Source: CAD feature listing. Evaluate the final solid. Frame: model axes, mm. Face numbers are marked on the shaded views. A direction names the side the tool comes from. Coordinates: 2 decimals unless noted, no trailing zeros. Loops run counter-clockwise (first coordinate to the right, second up) from the corner with the lowest first, then second, coordinate; pieces in that order, holes last.
Item 1: Line query: probe 1 along Y at (x, z) = (-23, 19); probe 2 along X at (y, z) = (54.5, 16.5); probe 3 along Z at (x, y) = (23, 43) (3 decimals). Output: solid intervals per line, ascending.
Item 2: Section query A-A, the plane z = 56.5. Return the cut outline in (x, y).
Item 3: Pull-direction query (X, two-part tool) for the marked faces 1, 2 and 3; classes: +X half, -X half, draft (parallel to the pull), parting line (faces both ways), or undercut.
Item 4: Section query C-C, the plane z = 19.05. Return the cut outline in (x, y), then the cut area to 3 significant figures.
Item 5: Reachability of the marked faces 4 and 5 from +Z, -Z, +X, -X, +Y, -Y: full face, straight path, thin tool, end or side. Return the list, or none.
Item 6: Pin query (flat end, axial travel): pin 1 Ø5 at (x, y) = (-11.5, 40) entering from -Z (3 decimals); pin 2 Ø12 at (y, z) = (19, 66.5) entering from -X; pin 3 Ø6 at (x, y) = (31.5, 56.5) entering from -Z. Return the tip coordinate at first contact, or that it passes through.
Item 7: Section query B-B, the plane y = 31.75. State how many separate pieces and enclosed holes the cut face has, then the cut area to 3 significant figures.
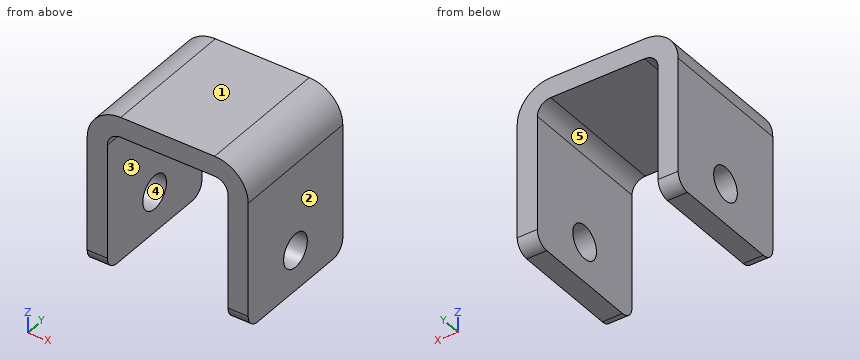
```python
from build123d import *

# Parameters (mm, degrees)
F0_W     = 76.2
F0_H     = 76.2
F1_DEPTH = 63.5
F2_T     = -9.525
F3_R     = 6.35
F4_R     = 15.875
F5_R     = 7.9375
F6_DEPTH = 76.201
F7_R     = 6.35


with BuildPart() as f1:
    # F0 (on Front) → F1 (new body)
    with BuildSketch(Plane.XZ):
        with Locations((7.4331681192, 38.1)):
            Rectangle(F0_W, F0_H)
    extrude(amount=-F1_DEPTH)

    # F2
    f2_openings = [f1.faces().sort_by_distance(p)[0] for p in [
        (7.433168, 0, 38.1),
        (7.433168, 31.75, 0),
        (7.433168, 63.5, 38.1),
    ]]
    offset(amount=F2_T, openings=f2_openings)

    # F3
    f3_edges = [f1.edges().sort_by_distance(p)[0] for p in [
        (-21.141832, 31.75, 66.675),
        (36.008168, 31.75, 66.675),
    ]]
    fillet(f3_edges, radius=F3_R)

    # F4
    f4_edges = [f1.edges().sort_by_distance(p)[0] for p in [
        (-30.666832, 31.75, 76.2),
        (45.533168, 31.75, 76.2),
    ]]
    fillet(f4_edges, radius=F4_R)

    # F5 (on face) → F6 (cut, through all)
    with BuildSketch(Plane.YZ.offset(45.5331681192)):
        with Locations((31.75, 19.05)):
            Circle(F5_R)
    extrude(amount=-F6_DEPTH, mode=Mode.SUBTRACT)

    # F7
    f7_edges = [f1.edges().sort_by_distance(p)[0] for p in [
        (-25.904332, 0, 0),
        (40.770668, 0, 0),
        (-25.904332, 63.5, 0),
        (40.770668, 63.5, 0),
    ]]
    fillet(f7_edges, radius=F7_R)


solid = f1.part
```
Verdict:
1. probe 1: y = 0 to 23.81, 39.69 to 63.5
1. probe 2: x = -30.67 to -21.14, 36.01 to 45.53
1. probe 3: z = 66.675 to 76.2
2. outline: (-30.67, 0) - (-21.14, 0) - (-21.14, 63.5) - (-30.67, 63.5) - close; (36.01, 0) - (45.53, 0) - (45.53, 63.5) - (36.01, 63.5) - close
3. face 1: draft
3. face 2: +X half
3. face 3: undercut
4. outline: (-30.67, 0) - (-21.14, 0) - (-21.14, 23.81) - (-30.67, 23.81) - close; (-30.67, 39.69) - (-21.14, 39.69) - (-21.14, 63.5) - (-30.67, 63.5) - close; (36.01, 0) - (45.53, 0) - (45.53, 23.81) - (36.01, 23.81) - close; (36.01, 39.69) - (45.53, 39.69) - (45.53, 63.5) - (36.01, 63.5) - close
4. area: 907 mm2
5. face 4: +X, -X
5. face 5: -Z, +Y, -Y
6. pin 1: stops at z = 66.675
6. pin 2: stops at x = -30.67
6. pin 3: stops at z = 64.43
7. separate pieces: 3
7. enclosed holes: 0
7. area: 1,600 mm2
